Geometry: see drawing. Coordinates: mm, zero at the bounding-box minimum. A direction names the side the tool comes from. Round coordinates to 2 decimals unless told otherwise and drop trailing zeros. Write each loop counter-clockwise with the first axis right and the second up, starting at its lowest first coordinate (ties: lowest second). Pieces come first, ordered by that corner, then holes. Notation, with made-up numbers: (21, 36) -> (67, 36) arc R21 ccw to (67, 60) -> close; hole circle Ø2 at (-10, 76). An arc over 180 degrees is marked (long way). Use CSV: the item, a comma, the result in double quotes.
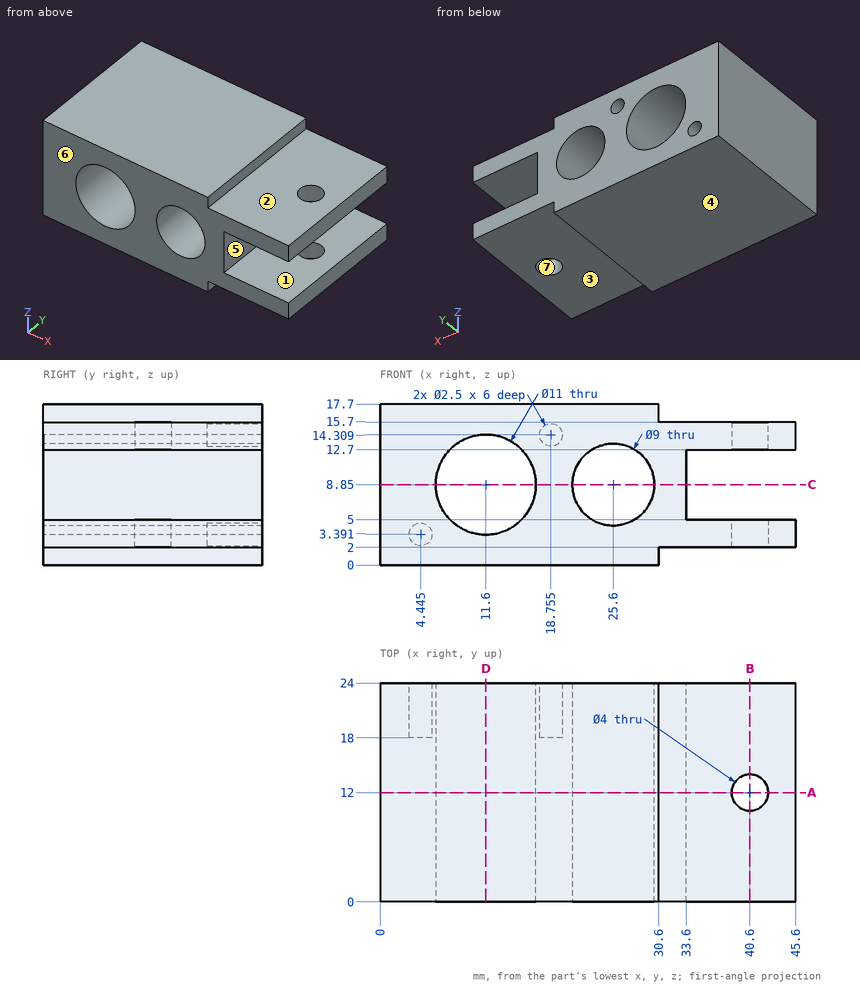
Item 1: Line query: line 1 (Z direction, x = 39, y = 2.5); line 2 (X direction, y = 12, z = 14.7); line 3 (Y direction, x = 40.6, z = 14.25). Output: solid intervals per line, ascending.
Worked answers:
line 1,"z = 2 to 5, 12.7 to 15.7"
line 2,"x = 0 to 38.6, 42.6 to 45.6"
line 3,"y = 0 to 10, 14 to 24"
Item 2: First-contact query: pin 1 Ø0.8 at (x, z) = (19, 15) entering from +Y; pin 2 Ø4.5 at (x, y) = (37, 16.5) entering from +Z; pin 3 Ø9 at (x, z) = (11.6, 8.85) entering from +Y; pin 4 Ø1 at (y, z) = (14.5, 16.5) entering from +X. Flat tips, straight axial feed; report the tip coordinate or a pass-through.
Worked answers:
pin 1,"stops at y = 18"
pin 2,"stops at z = 15.7"
pin 3,"passes through"
pin 4,"stops at x = 30.6"
Item 3: Section query D-D on x = 11.6. Return the cut outline in (y, z), plus the area to 3 significant figures.
Worked answers:
outline,"(0, 0) -> (24, 0) -> (24, 3.35) -> (0, 3.35) -> close; (0, 14.35) -> (24, 14.35) -> (24, 17.7) -> (0, 17.7) -> close"
area,"161 mm²"
Item 4: Set-up query: the marked faces 1, 2, 3 and 4. Return all of +Z, -Z, +X, -X, +Y, -Y with unobstructed straight access to the full face (end or side cutting, diameter ignored); none if empty.
Worked answers:
face 1,"+X, +Y, -Y"
face 2,"+Z, +X, +Y, -Y"
face 3,"-Z, +X, +Y, -Y"
face 4,"-Z, +X, -X, +Y, -Y"
Item 5: Section query A-A on y = 12. Return the cut outline in (x, z).
Worked answers:
outline,"(0, 0) -> (30.6, 0) -> (30.6, 2) -> (38.6, 2) -> (38.6, 5) -> (33.6, 5) -> (33.6, 12.7) -> (38.6, 12.7) -> (38.6, 15.7) -> (30.6, 15.7) -> (30.6, 17.7) -> (0, 17.7) -> close; (42.6, 2) -> (45.6, 2) -> (45.6, 5) -> (42.6, 5) -> close; (42.6, 12.7) -> (45.6, 12.7) -> (45.6, 15.7) -> (42.6, 15.7) -> close; hole circle Ø11 at (11.6, 8.85); hole circle Ø9 at (25.6, 8.85)"
Item 6: Section query B-B on x = 40.6. Return the cut outline in (y, z), plus the area to 3 significant figures.
Worked answers:
outline,"(0, 2) -> (10, 2) -> (10, 5) -> (0, 5) -> close; (0, 12.7) -> (10, 12.7) -> (10, 15.7) -> (0, 15.7) -> close; (14, 2) -> (24, 2) -> (24, 5) -> (14, 5) -> close; (14, 12.7) -> (24, 12.7) -> (24, 15.7) -> (14, 15.7) -> close"
area,"120 mm²"
Item 7: Section query C-C on z = 8.85. Return the cut outline in (x, y).
Worked answers:
outline,"(0, 0) -> (6.1, 0) -> (6.1, 24) -> (0, 24) -> close; (17.1, 0) -> (21.1, 0) -> (21.1, 24) -> (17.1, 24) -> close; (30.1, 0) -> (33.6, 0) -> (33.6, 24) -> (30.1, 24) -> close"
Item 8: Pull-direction query (X, two-part tool) for the marked faces 5, 6 and 7; classes: +X half, -X half, draft (parallel to the pull), parting line (faces both ways), or undercut.
Worked answers:
face 5,"+X half"
face 6,"draft"
face 7,"undercut"
